Input: part model. Units: mm. Frame: model coordinates. Face numbers are marked on the shaded views. A direction names the side the tool comes from. Round coordinates to 2 decimals unless told otherwise and drop trailing zeros. Loops run counter-clockwise (first coordinate to the right, second up) from the corner with the lowest first, then second, coordinate; pieces in that order, holes last.
(1) Access query for the marked faces 1, 2 and 3. Directions: +Z, -Z, +X, -X, +Y, -Y. A direction counts if a zero-diameter tool reaches every point of the face in a straight line with its end or side. Return the directions, or none.
(2) Line query: line 1 (Y direction, x = 5, z = 3.25); line 2 (X direction, y = 8.5, z = 6.5); line 3 (X direction, y = 9.5, z = 4.5). Output: solid intervals per line, ascending.
(3) Cut plane B-B, the plane x = 12. Output: boundary loops of the cut face in (y, z), and give its area (3 significant figures).
(4) Cut plane C-C, the plane z = 10. Output: boundary loops of the cut face in (x, y), and give its area (3 significant figures).
(5) First-contact query: pin 1 Ø4 at (y, z) = (8, 4.5) entering from +X; pin 2 Ø5 at (x, z) = (14.5, 10.5) entering from +Y; pin 3 Ø2.5 at (y, z) = (0.5, 8) entering from -X. Flat tips, straight axial feed; report the tip coordinate or a pass-through.
(6) Cut plane A-A, the plane y = 8.5. Output: boundary loops of the cut face in (x, z).
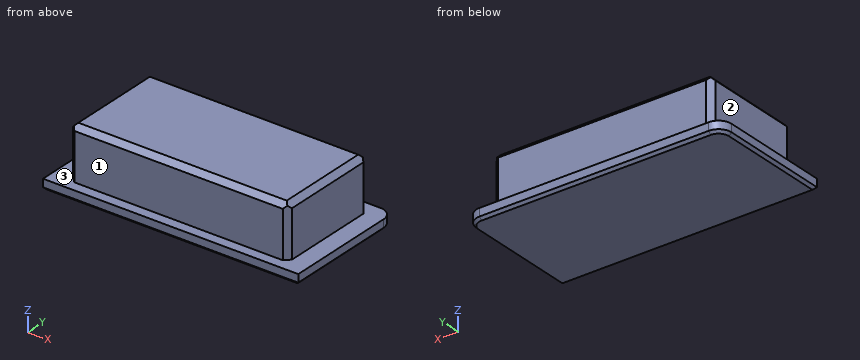
from build123d import *

# Parameters (mm, degrees)
SKETCH_W        = 49
SKETCH_H        = 24
PAD_DEPTH       = 2
SKETCH001_W     = 42
SKETCH001_H     = 20
PAD001_DEPTH    = 10
FILLET_R        = 2.5
CHAMFER_SIZE    = 1
CHAMFER001_SIZE = 1
CHAMFER002_SIZE = 0.5


with BuildPart() as part:
    # Sketch → Pad (new body)
    with BuildSketch(Plane.XY):
        Rectangle(SKETCH_W, SKETCH_H)
    extrude(amount=PAD_DEPTH)

    # Sketch001 (on Face6 of Pad) → Pad001 (join)
    with BuildSketch(Plane.XY.offset(2)):
        Rectangle(SKETCH001_W, SKETCH001_H)
    extrude(amount=PAD001_DEPTH)

    # Fillet
    fillet_edges = [part.edges().sort_by_distance(p)[0] for p in [
        (24.5, 12, 1),
        (-24.5, 12, 1),
    ]]
    fillet(fillet_edges, radius=FILLET_R)

    # Chamfer
    chamfer_edges = [part.edges().sort_by_distance(p)[0] for p in [
        (-21, 0, 12),
        (0, -10, 12),
        (21, 0, 12),
        (0, 10, 12),
    ]]
    chamfer(chamfer_edges, length=CHAMFER_SIZE)

    # Chamfer001
    chamfer001_edges = [part.edges().sort_by_distance(p)[0] for p in [
        (-21, -10, 6.5),
        (-21, 10, 6.5),
        (21, -10, 6.5),
        (21, 10, 6.5),
    ]]
    chamfer(chamfer001_edges, length=CHAMFER001_SIZE)

    # Chamfer002
    chamfer002_edges = [part.edges().sort_by_distance(p)[0] for p in [
        (0, 12, 0),
        (24.5, -1.25, 0),
        (23.767767, 11.267767, 0),
        (-23.767767, 11.267767, 0),
        (-24.5, -1.25, 0),
        (0, -12, 0),
    ]]
    chamfer(chamfer002_edges, length=CHAMFER002_SIZE)


solid = part.part
Reported:
1. face 1: +Z, +X, -X, -Y
1. face 2: +Z, -X, +Y, -Y
1. face 3: +Z
2. line 1: y = -10 to 10
2. line 2: x = -21 to 21
2. line 3: x = -20.5 to 20.5
3. outline: (-12, 0.5) - (-11.5, 0) - (11.5, 0) - (12, 0.5) - (12, 2) - (10, 2) - (10, 11) - (9, 12) - (-9, 12) - (-10, 11) - (-10, 2) - (-12, 2) - close
3. area: 247 mm2
4. outline: (-21, -9) - (-20, -10) - (20, -10) - (21, -9) - (21, 9) - (20, 10) - (-20, 10) - (-21, 9) - close
4. area: 838 mm2
5. pin 1: stops at x = 21
5. pin 2: stops at y = 10
5. pin 3: stops at x = -21
6. outline: (-24.5, 0.5) - (-24, 0) - (24, 0) - (24.5, 0.5) - (24.5, 2) - (21, 2) - (21, 11) - (20, 12) - (-20, 12) - (-21, 11) - (-21, 2) - (-24.5, 2) - close
